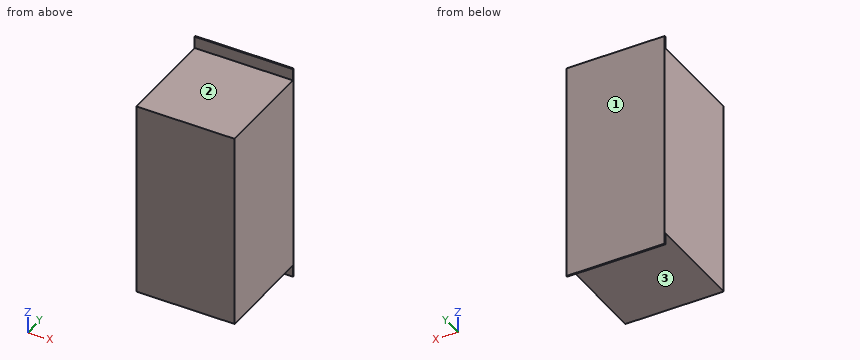
```python
from build123d import *

# Parameters (mm, degrees)
F0_W     = 231
F0_H     = 462
F1_DEPTH = 242
F0_H_2   = 28
F2_DEPTH = 3


with BuildPart() as f1:
    # F0 (on Front) → F1 (new body)
    with BuildSketch(Plane.XZ):
        Rectangle(F0_W, F0_H)
    extrude(amount=F1_DEPTH)

    # F0 (on Front) → F2 (join)
    with BuildSketch(Plane.XZ):
        with Locations((0, 245)):
            Rectangle(F0_W, F0_H_2)
        with Locations((0, -245)):
            Rectangle(F0_W, F0_H_2)
    extrude(amount=F2_DEPTH)


solid = f1.part
```
Work out the finished part from the listing and answer in its coordinate system (mm). Face numbers are marked on the shaded views. A direction names the side the tool comes from. Give positions to 0.01 mm unless a question says otherwise; leave off trailing zeros. Loops run counter-clockwise (first coordinate to the right, second up) from the corner with the lowest first, then second, coordinate; pieces in that order, holes last. Notation, with made-up numbers: (75, 23) -> (100, 23) arc R10 cw to (100, 28) -> close; hole circle Ø1 at (88.25, 58.25). An arc over 180 degrees is marked (long way). Write item = value, one per line. Start each with the question number.
(1) Given pin 1 Ø14 at (x, z) = (-23, 251) entering from -Y; pin 2 Ø6 at (x, y) = (-12, -167) entering from -Z, each flat-ended and moving along its own axis, determine where each tip first touches the part or whether it passes through.
(2) Find section B-B on y = -154. Give the vertices of the cut face in (x, z), and give its area (3 significant figures).
(3) Which of the six approach directions +Z, -Z, +X, -X, +Y, -Y give full straight-line access (tool end or side, diameter ignored) to the marked faces 1, 2 and 3?
(4) Find section A-A on x = 16.5. Give the vertices of the cut face in (y, z), and give its area (3 significant figures).
(5) Find the intervals of material crossed by probe 1 along Z at (x, y) = (-99, -110), in increasing order. Write a range as from..to.
From the geometry:
q1.pin_1 = -3
q1.pin_2 = -231
q2.outline = (-115.5, -231) -> (115.5, -231) -> (115.5, 231) -> (-115.5, 231) -> close
q2.area = 107,000 mm^2
q3.face_1 = +Z, -Z, +X, -X, +Y
q3.face_2 = +Z, +X, -X, -Y
q3.face_3 = -Z, +X, -X, -Y
q4.outline = (-242, -231) -> (-3, -231) -> (-3, -259) -> (0, -259) -> (0, 259) -> (-3, 259) -> (-3, 231) -> (-242, 231) -> close
q4.area = 112,000 mm^2
q5.probe_1 = -231..231
